Read the model definition and answer for the solid it produces. Units are mm, in the model's axes. A direction names the side the tool comes from. Coordinates: 2 decimals unless noted, no trailing zeros. Order: outer loops, then holes, each group sorted by start corner. A loop starts at its lowest first (then second) coordinate and runs counter-clockwise, first axis right, second up. Notation, with made-up numbers: M 33,-32.75 L 84,-32.75 A27 ccw 84,-11.75 Z; hole C -5,29.5 d2. An arc over 180 degrees is marked long. Use a Markdown table: item, result. Add a question column.
1) The mould has two halves that part along Z. Classify faces 1 (the face through (-31, 31, 50.8)), 2 (the face through (-17.1, -8.864, 26.689)), 3 (the face through (-62.293, 9, 25)), 4 (the face through (-4.84, 32.41, 6.13)): released by +Z, released by -Z, zero draft, split by the parting line, or undercut.
2) Find section A-A on z = 13.5. Write down the section's boundary in (x, y).
3) Find section B-B on y = -8.5. Count the separate pieces of the cut face and the enclosed holes in it, plus the area to 3 significant figures.
4) For faces 5 (the face through (-28, 8.293, 47)), 6 (the face through (-32, -33, 50.8)), determine the directions among +Z, -Z, +X, -X, +Y, -Y from which every point of the face is accessible in a straight line to the end or side of a thin tool.
5) Find section C-C on x = -51.5. Write down the section's boundary in (y, z), plus the area to 3 significant figures.
6) Each of these flat-tipped pins is pushed along its axis until it touches: pin 1 Ø13 at (y, z) = (35.06, 11.21) entering from +X; pin 2 Ø8 at (x, z) = (-38.5, 48.5) entering from -Y; pin 3 Ø10 at (x, z) = (-18.5, 15.5) entering from -Y. Where does it stop, or does it pass through?
7) Find section D-D on x = 43. Write down the section's boundary in (y, z).
8) Find the intervals of material crossed by probe 1 along Z at (x, y) = (-18.5, 35); probe 2 along Y at (x, z) = (-22.5, 29.5); probe 3 along Y at (x, z) = (-37.5, 11.5), in increasing order. Write a range as [from, to].
from build123d import *

# Parameters (mm, degrees)
F1_DEPTH  = 50.8
F3_DEPTH  = 0.189480841
F4_DEPTH  = 89.7186418795
F5_W      = 13.382118661
F5_H      = 7.166751343
F6_DEPTH  = 122.8903324733
F7_W      = 78.6715284359
F7_H      = 50.8
F8_DEPTH  = 25.4
F10_DEPTH = 25.4
F11_R     = 6.2312707334
F12_DEPTH = 122.8903324733
F13_R     = 6.1393781486
F14_DEPTH = 122.8903324733
F15_R     = 5.7324119576
F16_DEPTH = 122.8903324733
F17_R     = 5.5689542342
F18_DEPTH = 122.8903324733


with BuildPart() as f1:
    # F0 (on Top) → F1 (new body)
    with BuildSketch(Plane.XY):
        Polygon((-62.2928291559, 52.9630370438), (-62.2928291559, -36.376748234), (60.5965033174, -36.5652292967), (60.5965033174, 52.9630370438), align=None)
    extrude(amount=F1_DEPTH)

    # F2 (on face) → F3 (join, through all)
    with BuildSketch(Plane(origin=(-0.0559391088, -36.4722038357, 0), x_dir=(0.9999988238, -0.0015337445, 0), z_dir=(-0.0015337445, -0.9999988238, 0))):
        Polygon((60.6525137648, 50.8), (-0.7922247423, 50.8), (60.6525137648, 0), align=None)
    extrude(amount=F3_DEPTH)

    # F4 (cut, through all): a face of the model
    f4_faces = [f1.faces().sort_by_distance(p)[0] for p in [
        (40.1146572899, -36.7232964043, 33.8666666667),
    ]]
    extrude(f4_faces, amount=-F4_DEPTH, mode=Mode.SUBTRACT)

    # F5 (on face) → F6 (cut, through all)
    with BuildSketch(Plane(origin=(-62.2928291559, 0, 0), x_dir=(0, -1, 0), z_dir=(-1, 0, 0))):
        with Locations((-1.6020850744, 47.2166243285)):
            Rectangle(F5_W, F5_H)
    extrude(amount=-F6_DEPTH, mode=Mode.SUBTRACT)

    # F7 (on face) → F8 (join)
    with BuildSketch(Plane(origin=(-0.0559391088, -36.4722038357, 0), x_dir=(0.9999988238, -0.0015337445, 0), z_dir=(-0.0015337445, -0.9999988238, 0))):
        with Locations((-22.9011990315, 25.4)):
            Rectangle(F7_W, F7_H)
    extrude(amount=F8_DEPTH)

    # F9 (on face) → F10 (cut)
    with BuildSketch(Plane(origin=(-0.0948962197, -61.8721739606, 0), x_dir=(0.9999988238, -0.0015337445, 0), z_dir=(-0.0015337445, -0.9999988238, 0))):
        Polygon((16.4345651865, 50.8), (0, 50.8), (16.4345651865, 40.9449264407), align=None)
    extrude(amount=-F10_DEPTH, mode=Mode.SUBTRACT)

    # F11 (on face) → F12 (cut, through all)
    with BuildSketch(Plane(origin=(-62.2928291559, 0, 0), x_dir=(0, -1, 0), z_dir=(-1, 0, 0))):
        with Locations((-34.8689034581, 31.0050528497)):
            Circle(F11_R)
    extrude(amount=-F12_DEPTH, mode=Mode.SUBTRACT)

    # F13 (on face) → F14 (cut, through all)
    with BuildSketch(Plane(origin=(-62.2928291559, 0, 0), x_dir=(0, -1, 0), z_dir=(-1, 0, 0))):
        with Locations((6.031378638, 32.1359373629)):
            Circle(F13_R)
    extrude(amount=-F14_DEPTH, mode=Mode.SUBTRACT)

    # F15 (on face) → F16 (cut, through all)
    with BuildSketch(Plane(origin=(-62.2928291559, 0, 0), x_dir=(0, -1, 0), z_dir=(-1, 0, 0))):
        with Locations((-35.0573845208, 11.2145934254)):
            Circle(F15_R)
    extrude(amount=-F16_DEPTH, mode=Mode.SUBTRACT)

    # F17 (on face) → F18 (cut, through all)
    with BuildSketch(Plane(origin=(-62.2928291559, 0, 0), x_dir=(0, -1, 0), z_dir=(-1, 0, 0))):
        with Locations((5.6544179097, 11.5915555507)):
            Circle(F17_R)
    extrude(amount=-F18_DEPTH, mode=Mode.SUBTRACT)


solid = f1.part
Check result:
| question | item | result |
|---|---|---|
| 1 | face 1 | released by +Z |
| 1 | face 2 | undercut |
| 1 | face 3 | zero draft |
| 1 | face 4 | undercut |
| 2 | outline | M -62.33,-61.78 L 16.34,-61.9 L 16.38,-36.5 L 44.27,-36.54 L 44.31,-10.89 L -62.29,-10.89 L -62.29,-36.38 Z; M -62.29,-0.42 L 44.32,-0.42 L 44.37,29.8 L -62.29,29.8 Z; M -62.29,40.31 L 44.39,40.31 L 44.4,52.96 L -62.29,52.96 Z |
| 3 | separate pieces | 3 |
| 3 | enclosed holes | 0 |
| 3 | area | 2,700 mm2 |
| 4 | face 5 | +Z, +X, -X |
| 4 | face 6 | +Z, +X, -X, +Y, -Y |
| 5 | outline | M -61.79,0 L 52.96,0 L 52.96,50.8 L 8.29,50.8 L 8.29,43.63 L -5.09,43.63 L -5.09,50.8 L -61.79,50.8 Z; hole C -6.03,32.14 d12.28; hole C -5.65,11.59 d11.14; hole C 34.87,31.01 d12.46; hole C 35.06,11.21 d11.46 |
| 5 | area | 5,290 mm2 |
| 6 | pin 1 | stops at x = 55.01 |
| 6 | pin 2 | stops at y = -61.82 |
| 6 | pin 3 | stops at y = -61.85 |
| 7 | outline | M -36.54,0 L 52.96,0 L 52.96,14.66 L 39.65,14.64 A5.73 cw long 30.46,14.63 L -0.96,14.59 A5.57 cw long -10.35,14.58 L -36.54,14.55 Z |
| 8 | probe 1 | z = [0, 5.48], [16.95, 24.78], [37.23, 50.8] |
| 8 | probe 2 | y = [-61.84, -11.58], [-0.49, 28.82], [40.92, 52.96] |
| 8 | probe 3 | y = [-61.81, -11.22], [-0.09, 29.33], [40.78, 52.96] |
